Can you work these out from the model? Positions are in its coordinate system, mm. A direction names the side the tool comes from. Give positions to 0.01 mm unless a question says otherwise; leave off trailing zeros. Order: outer loops, then holes, each group sorted by start corner. A loop starts at its lowest first (then second) coordinate and runs counter-clockwise, first axis right, second up. Notation, with made-up numbers: (-18.5, 57.5) - (16.5, 57.5) arc R20 cw to (16.5, 72.5) - close; hole circle Ø2 at (31, 44.5). An arc over 180 degrees is marked (long way). Answer as CSV lines item,"result".
```python
from build123d import *

# Parameters (mm, degrees)
SKETCH2_W           = 75
SKETCH2_H           = 9
BOSS_EXTRUDE1_DEPTH = 26
BOSS_EXTRUDE2_DEPTH = 20
BOSS_EXTRUDE3_DEPTH = 4


with BuildPart() as part:
    # Sketch2 → Boss-Extrude1 (new, symmetric)
    with BuildSketch(Plane.XY):
        with Locations((0, -44.5)):
            Rectangle(SKETCH2_W, SKETCH2_H)
    extrude(amount=BOSS_EXTRUDE1_DEPTH, both=True)

    # Sketch2_4 → Boss-Extrude2 (add, symmetric)
    with BuildSketch(Plane.XY):
        with BuildLine():
            Line((-12, 0), (-20, 0))
            ThreePointArc((-20, 0), (-15.811388301, -12.247448714), (-5, -19.364916731))
            Line((-5, -19.364916731), (-5, -40))
            Line((-5, -40), (5, -40))
            Line((5, -40), (5, -19.364916731))
            ThreePointArc((5, -19.364916731), (15.811388301, -12.247448714), (20, 0))
            Line((20, 0), (12, 0))
            ThreePointArc((12, 0), (0, -12), (-12, 0))
        make_face()
    extrude(amount=BOSS_EXTRUDE2_DEPTH, both=True)

    # Sketch2_5 → Boss-Extrude3 (add, symmetric)
    with BuildSketch(Plane.XY):
        with BuildLine():
            Line((37.5, -40), (20, 0))
            ThreePointArc((20, 0), (15.811388301, -12.247448714), (5, -19.364916731))
            Line((5, -19.364916731), (5, -40))
            Line((5, -40), (37.5, -40))
        make_face()
        with BuildLine():
            ThreePointArc((-5, -19.364916731), (-15.811388301, -12.247448714), (-20, 0))
            Line((-20, 0), (-37.5, -40))
            Line((-37.5, -40), (-5, -40))
            Line((-5, -40), (-5, -19.364916731))
        make_face()
    extrude(amount=BOSS_EXTRUDE3_DEPTH, both=True)


solid = part.part
```
1) Which directions (+Z, -Z, +X, -X, +Y, -Y) give clear straight access to the entire face, cutting with the end or side of a thin tool? Please do faces 1 (the flat face through (17, -24, 4)), 2 (the flat face through (-18, -29, -4)), 3 (the flat face through (-1, -40, 22)), 4 (the flat face through (5, -30, -12)), 5 (the cylindrical face through (-16, -12, 12)).
Answer block:
face 1,"+Z, +X"
face 2,"-Z, -X"
face 3,"+Z"
face 4,"-Z, +X"
face 5,"+Z, -X"
2) I want a section at D-D on y = -16.5. Write out the boundary of the cut face in (x, z).
Answer block:
outline,"(-27.22, -4) - (-11.3, -4) - (-11.3, -20) - (11.3, -20) - (11.3, -4) - (27.22, -4) - (27.22, 4) - (11.3, 4) - (11.3, 20) - (-11.3, 20) - (-11.3, 4) - (-27.22, 4) - close"
3) I need wall thicknesses on line 1 along Y through (x, z) = (-25, -12); line 2 along Z through (x, y) = (27, -32.5); line 3 along Z through (x, y) = (12, -2.5). Which ranges of each line are inside material? Lowest first, please. Write a range as [from, to].
Answer block:
line 1,"[-49, -40]"
line 2,"[-4, 4]"
line 3,"[-20, 20]"
4) I want a section at C-C on y = -8.5. Write out the boundary of the cut face in (x, z).
Answer block:
outline,"(-23.72, -4) - (-18.1, -4) - (-18.1, -20) - (-8.47, -20) - (-8.47, 20) - (-18.1, 20) - (-18.1, 4) - (-23.72, 4) - close; (8.47, -20) - (18.1, -20) - (18.1, -4) - (23.72, -4) - (23.72, 4) - (18.1, 4) - (18.1, 20) - (8.47, 20) - close"
5) I want a section at B-B on z = 1. Write out the boundary of the cut face in (x, y).
Answer block:
outline,"(-37.5, -49) - (37.5, -49) - (37.5, -40) - (20, 0) - (12, 0) arc R12 cw to (-12, 0) - (-20, 0) - (-37.5, -40) - close"
6) I'm going to push flat-ended pins straight in: P1, Ø6, axis at x = 1, z = -14, coming from the +Y side; P2, Ø1, axis at y = -29.5, z = 11, coming from the -X side; P3, Ø4, axis at y = -17, z = 5, coming from the +X side. Where does each tip first touch, or does it pass through?
Answer block:
P1,"y = -11.31"
P2,"x = -5"
P3,"x = 28.2"
7) I want a section at A-A on x = 0. Write out the boundary of the cut face in (y, z), plus the area to 3 significant figures.
Answer block:
outline,"(-49, -26) - (-40, -26) - (-40, -20) - (-12, -20) - (-12, 20) - (-40, 20) - (-40, 26) - (-49, 26) - close"
area,"1,590 mm2"
8) If we mould it in two halves opening along Y, with no side actions, what happens to faces 6 (the flat face through (16, 0, 0)), 7 (the cylindrical face through (-16, -12, -12)), 8 (the flat face through (0, -20, 20))? For each: +Y half, -Y half, draft (parallel to the pull), parting line (faces both ways), or undercut.
Answer block:
face 6,"+Y half"
face 7,"undercut"
face 8,"draft"
